The drawing under review shows one solid part. Ordinate dimensions are in mm from its lowest x, y, z. Round coordinates to 2 decimals unless told otherwise and drop trailing zeros. Loops run counter-clockwise (first coordinate to the right, second up) from the corner with the lowest first, then second, coordinate; pieces in that order, holes last. Notation, with made-up numbers: M -14,-38 L 29,-38 A14 ccw 29,-13 Z; hole C 47,20 d10. An arc over 180 degrees is marked long. Use a Markdown table: item, result.
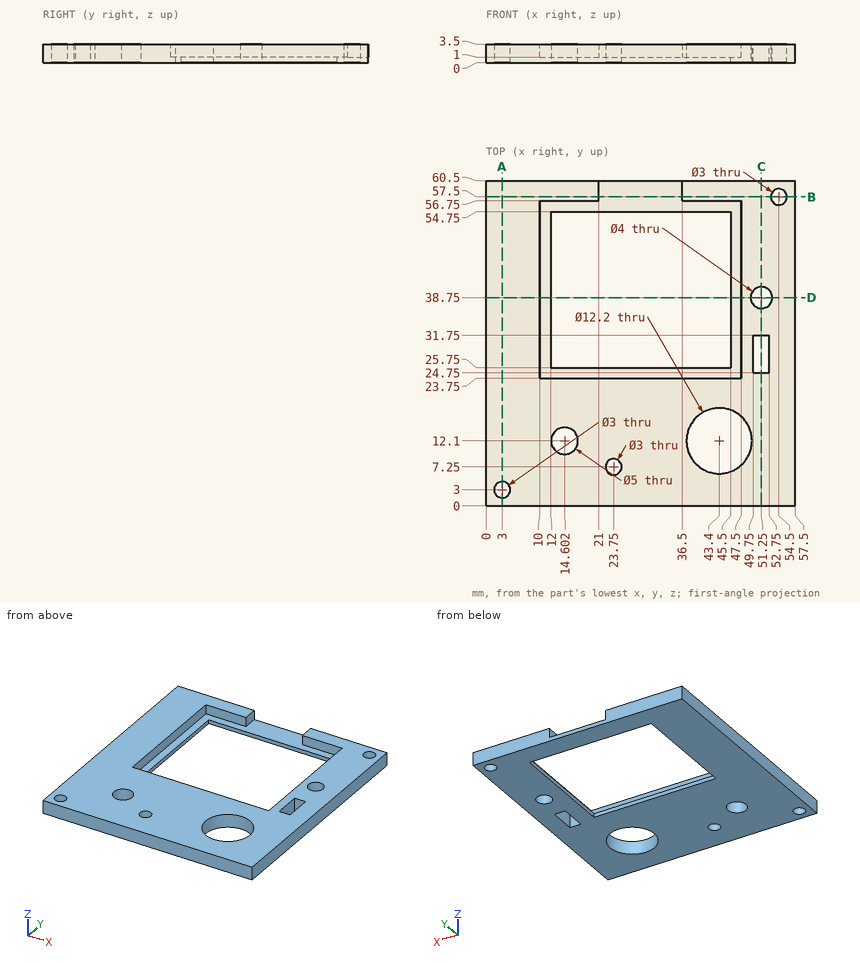
1. Insertion check: pin 1 (1.5 mm diameter, centred on x = 46, y = 51, fed in from +Z). The pin has a flat end and moves straight along its axis. Give the tip position at first contact, or say it passes through.
Check values:
| item | result |
|---|---|
| pin 1 | stops at z = 1 |
2. Take a section at A-A on x = 3. Give the boundary of the cut face in (y, z).
Check values:
| item | result |
|---|---|
| outline | M 0,0 L 1.5,0 L 1.5,3.5 L 0,3.5 Z; M 4.5,0 L 60.5,0 L 60.5,3.5 L 4.5,3.5 Z |
3. Take a section at B-B on y = 57.5. Give the boundary of the cut face in (x, z), and give its area (3 significant figures).
Check values:
| item | result |
|---|---|
| outline | M 0,0 L 53,0 L 53,3.5 L 36.5,3.5 L 36.5,1 L 21,1 L 21,3.5 L 0,3.5 Z; M 56,0 L 57.5,0 L 57.5,3.5 L 56,3.5 Z |
| area | 152 mm² |
4. Wall thickness on line 1 along Y through (x, z) = (43, 0.4); line 2 along Y through (x, z) = (54.5, 0.6); line 3 along X through (y, z) = (40.5, 1.4): over which ranges is each line inside the solid? List them lowest first. Write a range as from..to.
Check values:
| item | result |
|---|---|
| line 1 | y = 0..6.01, 18.19..25.75, 54.75..60.5 |
| line 2 | y = 0..56, 59..60.5 |
| line 3 | x = 0..10, 47.5..50.28, 52.22..57.5 |
5. Take a section at C-C on x = 51.25. Give the boundary of the cut face in (y, z), and give its area (3 significant figures).
Check values:
| item | result |
|---|---|
| outline | M 0,0 L 24.75,0 L 24.75,3.5 L 0,3.5 Z; M 31.75,0 L 36.75,0 L 36.75,3.5 L 31.75,3.5 Z; M 40.75,0 L 60.5,0 L 60.5,3.5 L 40.75,3.5 Z |
| area | 173 mm² |
6. Take a section at D-D on y = 38.75. Give the boundary of the cut face in (x, z).
Check values:
| item | result |
|---|---|
| outline | M 0,0 L 12,0 L 12,1 L 10,1 L 10,3.5 L 0,3.5 Z; M 45.5,0 L 49.25,0 L 49.25,3.5 L 47.5,3.5 L 47.5,1 L 45.5,1 Z; M 53.25,0 L 57.5,0 L 57.5,3.5 L 53.25,3.5 Z |
